Autodesk Inventor part; units mm, degrees
ref_plane "YZ Plane" through (0, 0, 0) normal (1, 0, 0) x (0, 1, 0)
ref_plane "XZ Plane" through (0, 0, 0) normal (0, 1, 0) x (-1, 0, 0)
ref_plane "XY Plane" through (0, 0, 0) normal (0, 0, 1) x (1, 0, 0)
sketch "草圖2" plane through (0, 0, 0) normal (0, 1, 0) x (-1, 0, 0)
  line L0 (10, 10) -> (-10, 10)
  line L1 (-10, 10) -> (-10, 0)
  line L2 (-10, -10) -> (0, -10) construction
  line L3 (10, -10) -> (10, 10)
  arc A0 (-10, 0) -> (0, -10) centre (0, 0) ccw
  line L4 (-10, 0) -> (-10, -10) construction
  line L5 (0, -10) -> (10, -10)
  circle A1 centre (0, 0) radius 5
  point P0 (0, 0)
  point P1 (10, 0)
  dimension "d2" = 20
  dimension "d3" = 20
  dimension "d4" = 10
  dimension "d5" = 10
  dimension "d6" = 10
extrude "擠出1" add sketch "草圖2" along normal blind 10
sketch "草圖3" plane through (-10, 0, 10) normal (0, 0, 1) x (1, 0, 0)
  line L0 (0, 10) -> (20, 10)
  line L1 (20, 10) -> (15, 15)
  line L2 (15, 15) -> (10, 15)
  line L3 (10, 15) -> (5, 20)
  line L4 (5, 20) -> (0, 20)
  line L5 (0, 20) -> (0, 10)
  point P0 (10, 0)
  dimension "d9" = 5
  dimension "d10" = 5
  dimension "d11" = 5
  dimension "d12" = 5
  dimension "d13" = 10
extrude "擠出2" add sketch "草圖3" against normal blind 5
sketch "草圖4" plane through (-10, 0, -10) normal (-1, 0, 0) x (0, 0, 1)
  line L0 (15, 10) -> (15, 20)
  line L1 (15, 20) -> (10, 15)
  line L2 (10, 15) -> (10, 10)
  line L3 (10, 0) -> (10, 10)
  line L4 (15, 10) -> (10, 10)
  dimension "d16" = 5
  dimension "d17" = 5
extrude "擠出3" add sketch "草圖4" against normal blind 5
sketch "草圖5" plane through (0, 10, 0) normal (0, 1, 0) x (1, 0, 0)
  line L0 (-10, 10) -> (-5, 10)
  line L1 (-5, 10) -> (-5, 5)
  line L2 (-5, 5) -> (-10, 5)
  line L3 (-10, 5) -> (-10, 10)
  line L4 (-5, 0) -> (-5, -5)
  point P0 (0, 0)
  dimension "d20" = 5
  dimension "d21" = 5
extrude "擠出4" add sketch "草圖5" along normal blind 5
properties part number "20"
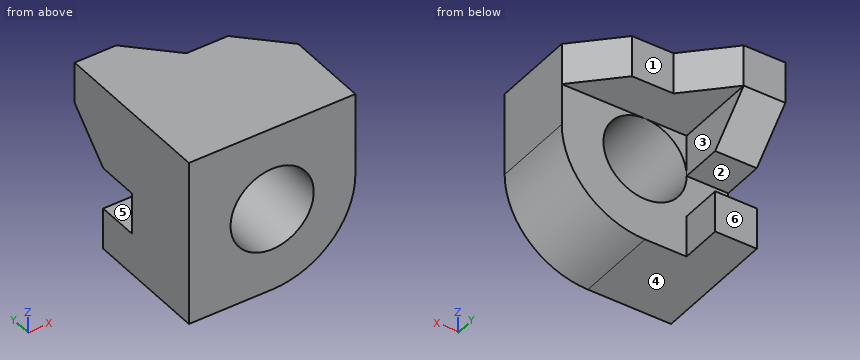
Check sheet for the modelled part. Datum: model origin and axes. Units: mm. Face numbers are marked on the shaded views. A direction names the side the tool comes from. Round coordinates to 2 decimals unless told otherwise and drop trailing zeros. Loops run counter-clockwise (first coordinate to the right, second up) from the corner with the lowest first, then second, coordinate; pieces in that order, holes last. Notation, with made-up numbers: (-31, -35.5) - (23, -35.5) arc R19 cw to (23, -13.5) - close; hole circle Ø4 at (-17.5, -34.5). An arc over 180 degrees is marked (long way). Answer as a JSON object with one key per item and string values. Group by question number.
Q1. Mould release check, pull along Z, two halves, no side actions. Record for the marked faces 4, 5 and 6: released by +Z, released by -Z, zero draft, split by the parting line, or undercut.
Q2. Sectioned sample at D-D, the plane x = -8.5. Enter the section's corners in (y, z).
Q3. Set-up check for the marked faces 1, 2 and 3: record each of +Z, -Z, +X, -X, +Y, -Y from which the full face is reachable in a straight line by a thin tool's end or side.
Q4. Gauge pin test, flat ends, axial feed: P1, Ø1.5, axis at y = 13.5, z = -8, coming from the +X side; P2, Ø12, axis at x = 2, z = -3, coming from the +Y side; P3, Ø5, axis at x = 6, y = 15.5, coming from the -Z side; P4, Ø1.5, axis at x = -1.5, z = 2, coming from the +Y side. Record the tip position at first contact, or that the pin passes through.
Q5. Sectioned sample at A-A, the plane x = -4. Enter the section's corners in (y, z), plus the area to 3 significant figures.
Q6. Sectioned sample at B-B, the plane z = 1.75. Enter the section's corners in (x, y).
Q7. Scan lines: line 1 along X through (y, z) = (4.25, 0); line 2 along Y through (x, z) = (5.25, -4.5). Record each from-to range of solid material in increasing order. Write a range as [from, to].
Q8. Sectioned sample at C-C, the plane y = 17.75. Enter the section's corners in (x, z).
Solution:
{
 "1": {"face 4": "released by -Z", "face 5": "undercut", "face 6": "zero draft"},
 "2": {"outline": "(0, -10) - (15, -10) - (15, -5) - (10, -5) - (10, 0) - (15, 0) - (20, 5) - (20, 10) - (0, 10) - close"},
 "3": {"face 1": "+Z, -Z, +X, +Y", "face 2": "+X, -X, +Y", "face 3": "-Z, +X, +Y"},
 "4": {"P1": "stops at x = -5", "P2": "stops at y = 10", "P3": "stops at z = 5", "P4": "passes through"},
 "5": {"outline": "(0, -10) - (10, -10) - (10, -3) - (0, -3) - close; (0, 3) - (10, 3) - (10, 5) - (19, 5) - (19, 10) - (0, 10) - close", "area": "185 mm²"},
 "6": {"outline": "(-10, 0) - (-4.68, 0) - (-4.68, 10) - (-5, 10) - (-5, 16.75) - (-10, 16.75) - close; (4.68, 0) - (10, 0) - (10, 10) - (4.68, 10) - close"},
 "7": {"line 1": "x = [-10, -5], [5, 10]", "line 2": "y = [0, 10]"},
 "8": {"outline": "(-10, 2.75) - (-5, 2.75) - (-5, 5) - (-2.75, 5) - (-2.75, 10) - (-10, 10) - close"}
}
